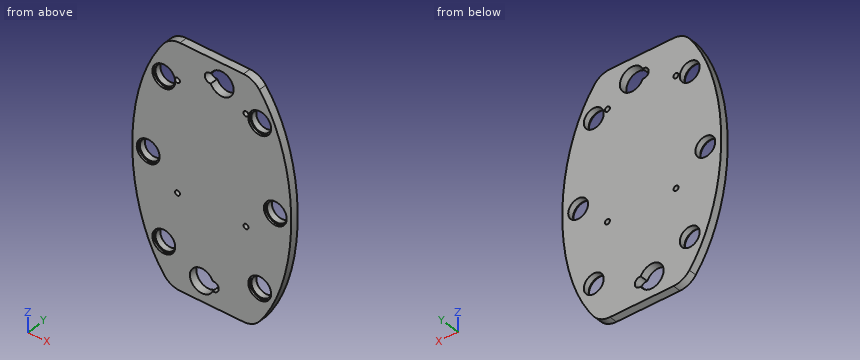
from build123d import *

# Parameters (mm, degrees)
SKETCH1_R           = 5
BOSS_EXTRUDE1_DEPTH = 4
SKETCH3_R           = 5.75
CUT_EXTRUDE2_DEPTH  = 1
CUT_EXTRUDE3_REACH  = 74.222
SKETCH4_R           = 1.25


with BuildPart() as part:
    # Sketch1 → Boss-Extrude1 (new body)
    with BuildSketch(Plane(origin=(0, 0, 0), x_dir=(1, 0, 0), z_dir=(0, 1, 0))):
        with BuildLine():
            Line((-15.999553812, 60), (15.999553812, 60))
            ThreePointArc((15.999553812, 60), (20.429760931, 58.965113769), (23.94301598, 56.074652977))
            add(Edge.make_bspline(
                [(23.94301598, -56.074652977), (66.825332337, 0), (23.94301598, 56.074652977)],
                knots=[3.783314198, 3.783314198, 3.783314198, 5.641463762, 5.641463762, 5.641463762], degree=2, weights=[1, 0.598575399, 1]))
            ThreePointArc((23.94301598, -56.074652977), (20.429760931, -58.965113769), (15.999553812, -60))
            Line((15.999553812, -60), (-15.999553812, -60))
            ThreePointArc((-15.999553812, -60), (-20.429760931, -58.965113769), (-23.94301598, -56.074652977))
            add(Edge.make_bspline(
                [(-23.94301598, 56.074652977), (-66.825332337, 0), (-23.94301598, -56.074652977)],
                knots=[0.641721545, 0.641721545, 0.641721545, 2.499871109, 2.499871109, 2.499871109], degree=2, weights=[1, 0.598575399, 1]))
            ThreePointArc((-23.94301598, 56.074652977), (-20.429760931, 58.965113769), (-15.999553812, 60))
        make_face()
        with Locations(Location((-32, 0, 0), (0, 0, 270))):
            Circle(SKETCH1_R, mode=Mode.SUBTRACT)
        with Locations(Location((-24.141452548, 40, 0), (0, 0, 270))):
            Circle(SKETCH1_R, mode=Mode.SUBTRACT)
        with Locations(Location((-24.141452548, -40, 0), (0, 0, 270))):
            Circle(SKETCH1_R, mode=Mode.SUBTRACT)
        with Locations(Location((24.141452548, -40, 0), (0, 0, 90))):
            Circle(SKETCH1_R, mode=Mode.SUBTRACT)
        with Locations(Location((32, 0, 0), (0, 0, 90))):
            Circle(SKETCH1_R, mode=Mode.SUBTRACT)
        with Locations(Location((24.141452548, 40, 0), (0, 0, 90))):
            Circle(SKETCH1_R, mode=Mode.SUBTRACT)
        with BuildLine():
            ThreePointArc((-0.479166667, -52.445144707), (11, -50), (-0.479166667, -47.554855293))
            ThreePointArc((-0.479166667, -47.554855293), (-3.5, -50), (-0.479166667, -52.445144707))
        make_face(mode=Mode.SUBTRACT)
        with BuildLine():
            ThreePointArc((0.479166667, 52.445144707), (-11, 50), (0.479166667, 47.554855293))
            ThreePointArc((0.479166667, 47.554855293), (3.5, 50), (0.479166667, 52.445144707))
        make_face(mode=Mode.SUBTRACT)
    extrude(amount=BOSS_EXTRUDE1_DEPTH)

    # Sketch3 → Cut-Extrude2 (cut)
    with BuildSketch(Plane.XZ):
        with Locations(Location((-24.141452548, -40, 0), (0, 0, 270))):
            Circle(SKETCH3_R)
        with Locations(Location((24.141452548, -40, 0), (0, 0, 270))):
            Circle(SKETCH3_R)
        with Locations(Location((32, 0, 0), (0, 0, 270))):
            Circle(SKETCH3_R)
        with Locations(Location((24.141452548, 40, 0), (0, 0, 270))):
            Circle(SKETCH3_R)
        with Locations(Location((-24.141452548, 40, 0), (0, 0, 270))):
            Circle(SKETCH3_R)
        with Locations(Location((-32, 0, 0), (0, 0, 270))):
            Circle(SKETCH3_R)
    extrude(amount=-CUT_EXTRUDE2_DEPTH, mode=Mode.SUBTRACT)

    # Sketch4 → Cut-Extrude3 (cut, up to next)
    with BuildSketch(Plane(origin=(0, 4, 0), x_dir=(1, 0, 0), z_dir=(0, 1, 0)), mode=Mode.PRIVATE) as cut_extrude3_sk1:
        with Locations(Location((17.25, -41.25, 0), (0, 0, 270))):
            Circle(SKETCH4_R)
    cut_extrude3_tool1 = extrude(cut_extrude3_sk1.sketch, amount=-CUT_EXTRUDE3_REACH, mode=Mode.PRIVATE) & part.part
    # Sketch4 → Cut-Extrude3 (cut, up to next)
    with BuildSketch(Plane(origin=(0, 4, 0), x_dir=(1, 0, 0), z_dir=(0, 1, 0)), mode=Mode.PRIVATE) as cut_extrude3_sk2:
        with Locations(Location((17.25, 13.25, 0), (0, 0, 270))):
            Circle(SKETCH4_R)
    cut_extrude3_tool2 = extrude(cut_extrude3_sk2.sketch, amount=-CUT_EXTRUDE3_REACH, mode=Mode.PRIVATE) & part.part
    # Sketch4 → Cut-Extrude3 (cut, up to next)
    with BuildSketch(Plane(origin=(0, 4, 0), x_dir=(1, 0, 0), z_dir=(0, 1, 0)), mode=Mode.PRIVATE) as cut_extrude3_sk3:
        with Locations(Location((-17.25, 13.25, 0), (0, 0, 270))):
            Circle(SKETCH4_R)
    cut_extrude3_tool3 = extrude(cut_extrude3_sk3.sketch, amount=-CUT_EXTRUDE3_REACH, mode=Mode.PRIVATE) & part.part
    # Sketch4 → Cut-Extrude3 (cut, up to next)
    with BuildSketch(Plane(origin=(0, 4, 0), x_dir=(1, 0, 0), z_dir=(0, 1, 0)), mode=Mode.PRIVATE) as cut_extrude3_sk4:
        with Locations(Location((-17.25, -41.25, 0), (0, 0, 270))):
            Circle(SKETCH4_R)
    cut_extrude3_tool4 = extrude(cut_extrude3_sk4.sketch, amount=-CUT_EXTRUDE3_REACH, mode=Mode.PRIVATE) & part.part
    add(cut_extrude3_tool1.solids().sort_by_distance((17.25, 4, 41.25))[0], mode=Mode.SUBTRACT)
    add(cut_extrude3_tool2.solids().sort_by_distance((17.25, 4, -13.25))[0], mode=Mode.SUBTRACT)
    add(cut_extrude3_tool3.solids().sort_by_distance((-17.25, 4, -13.25))[0], mode=Mode.SUBTRACT)
    add(cut_extrude3_tool4.solids().sort_by_distance((-17.25, 4, 41.25))[0], mode=Mode.SUBTRACT)


solid = part.part
Here's how the part is built. I have some questions about the finished solid (model axes, mm). Give positions to 0.01 mm unless a question says otherwise; leave off trailing zeros. Loops run counter-clockwise (first coordinate to the right, second up) from the corner with the lowest first, then second, coordinate; pieces in that order, holes last. Notation, with made-up numbers: (-12.75, 85.25) -> (42.25, 85.25) arc R28 ccw to (42.25, 104.25) -> close; hole circle Ø7 at (79.5, 45.5). An arc over 180 degrees is marked (long way). Answer as a JSON object with one key per item and string values. Group by question number.
Item 1: I need wall thicknesses on L1, parallel to Z at x = -16.5, y = 3.7; L2, parallel to Z at x = -23, y = 3.1; L3, parallel to Z at x = -4.5, y = 3.55. Which ranges of each line are inside material? Lowest first, please.
Item 2: Imagine slicing it at B-B on z = 0. Give the number of separate pieces and of enclosed holes in the cut face, then the cut area to 3 significant figures.
Item 3: Imagine slicing it at A-A on x = 5. Write out the boundary of the cut face in (y, z).
Item 4: Will these pins go through, and if not, where does the flat tip stop? pin 1 (2 mm diameter, centred on x = -28.5, y = 3, fed in from +Z); pin 2 (2 mm diameter, centred on y = 3, z = -30.5, fed in from -X).
Answer list:
{
 "1": {"L1": "z = -59.99 to -14.25, -12.25 to 40.25, 42.25 to 59.99", "L2": "z = -57.14 to -44.87, -35.13 to 35.13, 44.87 to 57.14", "L3": "z = -60 to -55.98, -44.02 to 60"},
 "2": {"separate pieces": "3", "enclosed holes": "0", "area": "237 mm2"},
 "3": {"outline": "(0, -60) -> (4, -60) -> (4, 44) -> (0, 44) -> close; (0, 56) -> (4, 56) -> (4, 60) -> (0, 60) -> close"},
 "4": {"pin 1": "stops at z = 50.83", "pin 2": "stops at x = -36.27"}
}
